Source: CAD feature listing. Evaluate the final solid. Frame: model axes, mm. Face numbers are marked on the shaded views. A direction names the side the tool comes from. Give positions to 0.01 mm unless a question says otherwise; leave off trailing zeros. Use CSV: the item, a comma, the result in double quotes. Start each with the question number.
Item 1: Access query for the marked faces 1 and 2. Directions: +Z, -Z, +X, -X, +Y, -Y. A direction counts if a zero-diameter tool reaches every point of the face in a straight line with its end or side. Return the directions, or none.
Item 2: Ray query, probe 1 along Y at (x, z) = (-58, -172); probe 2 along Z at (x, y) = (-79, 47.5); probe 3 along X at (y, z) = (95, -8.5). Return the intervals inside material, ascending. Write a range as from..to.
Item 3: First-contact query: pin 1 (10 mm diameter, centred on x = -156, z = -152.5, fed in from +Y); pin 2 (10 mm diameter, centred on x = -202.5, y = 77, fed in from +Z); pin 3 (8 mm diameter, centred on y = 36.5, z = -42, fed in from -X); pin 4 (1 mm diameter, centred on y = 35, z = -182, fed in from -X). Flat tips, straight axial feed; report the tip coordinate or a pass-through.
from build123d import *

# Parameters (mm, degrees)
ASPA_DEPTH          = 100
BOSS_EXTRUDE1_DEPTH = 3


with BuildPart() as part:
    # Sketch1 → Aspa (new body)
    with BuildSketch(Plane(origin=(0, 0, 0), x_dir=(1, 0, 0), z_dir=(0, 1, 0))):
        with BuildLine():
            ThreePointArc((25.447793126, 0.386570406), (24.230286438, -1.604077093), (22.239638939, -0.386570406))
            add(Edge.make_bspline(
                [(22.239638939, -0.386570406), (21.757478048, 1.614160196), (20.749121719, 5.597302334), (18.536030085, 13.574591529), (14.168694774, 27.479743189), (6.550840337, 47.079936231), (-4.628442304, 69.734907552), (-21.975568559, 98.239463115), (-47.651343304, 129.677792921), (-82.591872401, 157.938934972), (-112.981407164, 171.898903888), (-136.706178937, 176.753073489), (-153.882706061, 177.19977096), (-170.139849975, 174.457544689), (-182.693050278, 169.564346219), (-192.015134762, 164.134990799), (-198.616330487, 159.32363019), (-203.771296986, 154.710229964), (-207.666830265, 150.676861459), (-209.548220456, 148.533756447), (-210.459571896, 147.44572479)],
                knots=[1.285391812, 1.285391812, 1.285391812, 1.285391812, 1.319128815, 1.352865818, 1.420339824, 1.555287836, 1.690235848, 1.82518386, 2.095079884, 2.364975908, 2.634871932, 2.769819944, 2.904767956, 3.039715967, 3.174663979, 3.242137985, 3.309611991, 3.377085997, 3.410823, 3.444560003, 3.444560003, 3.444560003, 3.444560003], degree=3))
            ThreePointArc((-210.459571896, 147.44572479), (-212.783966565, 147.240324157), (-212.989367198, 149.564718827))
            add(Edge.make_bspline(
                [(25.447793126, 0.386570406), (24.469423216, 4.446324434), (22.333224695, 12.496143625), (17.278981997, 28.592037716), (9.575585068, 48.408864531), (-1.732113789, 71.325665764), (-19.282855172, 100.164756936), (-45.285499338, 132.010247367), (-80.787938764, 160.741243667), (-111.866153701, 175.039124584), (-136.310465657, 180.046556902), (-154.101500744, 180.513328396), (-171.016980761, 177.663303296), (-184.108550637, 172.560778181), (-193.824522276, 166.901653535), (-200.696906081, 161.892236402), (-206.053892172, 157.097615744), (-210.09605989, 152.912239242), (-212.044923282, 150.692258471), (-212.989367198, 149.564718827)],
                knots=[1.285391812, 1.285391812, 1.285391812, 1.285391812, 1.352865818, 1.420339824, 1.555287836, 1.690235848, 1.82518386, 2.095079884, 2.364975908, 2.634871932, 2.769819944, 2.904767956, 3.039715967, 3.174663979, 3.242137985, 3.309611991, 3.377085997, 3.410823, 3.444560003, 3.444560003, 3.444560003, 3.444560003], degree=3))
        make_face()
    extrude(amount=ASPA_DEPTH)

    # Sketch1<6> → Boss-Extrude1 (add)
    with BuildSketch(Plane(origin=(0, 0, 0), x_dir=(1, 0, 0), z_dir=(0, 1, 0))):
        with BuildLine():
            ThreePointArc((53.008754094, 7.028552828), (30.87226886, -29.165038062), (-5.321322029, -7.028552828))
            add(Edge.make_bspline(
                [(-5.321322029, -7.028552828), (-5.752950613, -5.237506451), (-6.655037469, -1.674110926), (-8.6398779, 5.480878278), (-11.443110905, 14.40659541), (-15.310525869, 25.045167991), (-21.110443607, 39.04951786), (-29.511654733, 56.07370943), (-45.107779267, 81.696632202), (-67.97631331, 109.640843996), (-98.089242139, 133.864294121), (-122.562455739, 144.921585832), (-140.105714345, 148.459050781), (-152.003061212, 148.733301905), (-162.60449903, 146.917163479), (-170.532615395, 143.822271696), (-176.470851118, 140.366842739), (-180.742294705, 137.256967741), (-184.161729253, 134.200415757), (-186.797539391, 131.472934141), (-188.099273447, 129.990261782), (-188.726330433, 129.241639658)],
                knots=[1.285391812, 1.285391812, 1.285391812, 1.285391812, 1.319128815, 1.352865818, 1.420339824, 1.48781383, 1.555287836, 1.690235848, 1.82518386, 2.095079884, 2.364975908, 2.634871932, 2.769819944, 2.904767956, 3.039715967, 3.174663979, 3.242137985, 3.309611991, 3.377085997, 3.410823, 3.444560003, 3.444560003, 3.444560003, 3.444560003], degree=3))
            ThreePointArc((-188.726330433, 129.241639658), (-230.988051698, 125.507082694), (-234.722608661, 167.768803959))
            add(Edge.make_bspline(
                [(53.008754094, 7.028552828), (51.929817399, 11.505609563), (49.571841508, 20.39092904), (44.012354136, 38.093264581), (35.556422664, 59.844015849), (23.1511521, 84.986891525), (3.849324765, 116.707571722), (-24.960519687, 152.047203238), (-65.290568749, 184.815877475), (-102.285114039, 202.016459154), (-132.910914262, 208.340551294), (-155.981206852, 208.979905408), (-178.552102656, 205.203280991), (-199.813171225, 196.924192445), (-215.737282567, 186.496778707), (-227.077525578, 176.342226424), (-232.269234058, 170.69780491), (-234.722608661, 167.768803959)],
                knots=[1.285391812, 1.285391812, 1.285391812, 1.285391812, 1.352865818, 1.420339824, 1.555287836, 1.690235848, 1.82518386, 2.095079884, 2.364975908, 2.634871932, 2.769819944, 2.904767956, 3.039715967, 3.174663979, 3.309611991, 3.377085997, 3.444560003, 3.444560003, 3.444560003, 3.444560003], degree=3))
        make_face()
    extrude(amount=-BOSS_EXTRUDE1_DEPTH)


solid = part.part
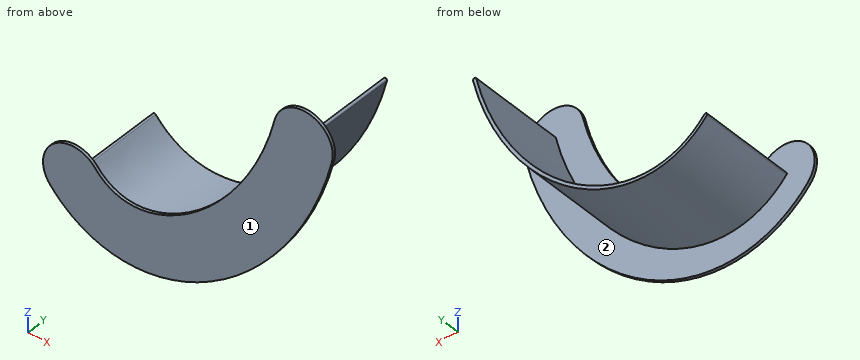
Verdict:
1,face 1,"+Z, -Z, +X, -X, -Y"
1,face 2,"+Y"
2,probe 1,"-3..0"
2,probe 2,"-157.48..-153.52"
2,probe 3,"19.94..23.36"
3,pin 1,"y = 0"
3,pin 2,"z = -150.81"
3,pin 3,"x = 6.62"
3,pin 4,"through"
